Here's how the part is built. I have some questions about the finished solid (model axes, mm). A direction names the side the tool comes from. Coordinates: 2 decimals unless noted, no trailing zeros. Order: outer loops, then holes, each group sorted by start corner. A loop starts at its lowest first (then second) coordinate and runs counter-clockwise, first axis right, second up. Notation, with made-up numbers: (12.5, 35.5) - (42.5, 35.5) arc R16 ccw to (42.5, 44.5) - close; hole circle Ø9 at (-3, 47). An arc over 180 degrees is marked (long way). Answer as CSV lines item,"result". Start each with the question number.
Q1. I need wall thicknesses on line 1 (Y direction, x = 26.5, z = 4); line 2 (X direction, y = 78, z = 1.15); line 3 (Y direction, x = 86, z = 4). Which ranges of each line are inside material? Lowest first, please.
Q2. Suppose I cut it at A-A (x = 50). Please give me the cut outline in (y, z), then the cut area to 4 significant figures.
Q3. For pin 1 Ø2.5 at (y, z) = (35.5, 3.5) entering from +X; pin 2 Ø2.5 at (y, z) = (37.5, 1.5) entering from -X; pin 3 Ø1 at (x, z) = (-26.5, 3.5) entering from -Y, each with a flat end and sliding along its axis, tell me the tip position at first contact or that it passes through.
Q4. Suppose I cut it at B-B (y = -114.5). Please give me the cut outline in (x, z), then the cut area to 3 significant figures.
Q5. Suppose I cut it at D-D (z = 3.95). Count the separate pieces of the cut face and the enclosed holes in it, then the cut area to 3 significant figures.
Q6. For faces 1 (the face through (-3, -86, 0)), 2 (the face through (-78, -44, 3)), 3 (the face through (-67.3, -102.615, 2.535)), which set-ups out of +Z, -Z, +X, -X, +Y, -Y let a thin tool reach every point of the face, with its end or its side?
Q7. Suppose I cut it at C-C (y = -141.5). Please give me the cut outline in (x, z), then the cut area to 3 significant figures.
Q8. Thinking about a two-plate mould opening in X: for faces 4 (the face through (226.035, -75.128, 2.465)), 5 (the face through (67.15, -102.48, 2.54)), 6 (the face through (-225.212, -72.74, 2.465)), which applies, released by +X, released by -X, zero draft, split by the parting line, or undercut?
from build123d import *

# Parameters (mm, degrees)
EXTRUDE_1_OUTLINE_R = 6.05
EXTRUDE_1_DEPTH     = 5
SKETCH_3_R          = 21.1
CUT_EXTRUDE_2_DEPTH = 281.223125384
FILLET_1_R          = 10
FILLET1_R           = 10
CUT_EXTRUDE1_DEPTH  = 10
FILLET2_R           = 5


# Read off the part's stored shape, not the designer's step: 凸台-拉伸1
with BuildPart() as part:
    # 凸台-拉伸1 outline → 凸台-拉伸1 (new body)
    with BuildSketch(Plane.XY):
        with BuildLine():
            ThreePointArc((-97.084973779, -160), (-77.084973779, -132.915026221), (-70, -100))
            Line((-70, -100), (70, -100))
            ThreePointArc((70, -100), (77.084973779, -132.915026221), (97.084973779, -160))
            Line((97.084973779, -160), (202.915026221, -160))
            ThreePointArc((202.915026221, -160), (224.833147735, -71.715728753), (150, -20))
            Line((150, -20), (150, 100))
            Line((150, 100), (-150, 100))
            Line((-150, 100), (-150, -20))
            ThreePointArc((-150, -20), (-224.833147735, -71.715728753), (-202.915026221, -160))
            Line((-202.915026221, -160), (-97.084973779, -160))
        make_face()
        with Locations((-50, -80)):
            Circle(EXTRUDE_1_OUTLINE_R, mode=Mode.SUBTRACT)
        with Locations((50, -80)):
            Circle(EXTRUDE_1_OUTLINE_R, mode=Mode.SUBTRACT)
        with Locations((-130, 0)):
            Circle(EXTRUDE_1_OUTLINE_R, mode=Mode.SUBTRACT)
        with Locations((-130, 79.62392947)):
            Circle(EXTRUDE_1_OUTLINE_R, mode=Mode.SUBTRACT)
        with Locations((130, 0)):
            Circle(EXTRUDE_1_OUTLINE_R, mode=Mode.SUBTRACT)
        with Locations((130, 80)):
            Circle(EXTRUDE_1_OUTLINE_R, mode=Mode.SUBTRACT)
    extrude(amount=EXTRUDE_1_DEPTH)

    # 草图3 → 切除-拉伸2 (cut, through all)
    with BuildSketch(Plane.XY.offset(5)):
        with Locations((-150, -100)):
            Circle(SKETCH_3_R)
        with Locations((150, -100)):
            Circle(SKETCH_3_R)
    extrude(amount=-CUT_EXTRUDE_2_DEPTH, mode=Mode.SUBTRACT)

    # 圆角1
    fillet_1_edges = [part.edges().sort_by_distance(p)[0] for p in [
        (-150, -20, 2.5),
        (-150, 100, 2.5),
        (150, 100, 2.5),
        (150, -20, 2.5),
        (70, -100, 2.5),
        (-70, -100, 2.5),
    ]]
    fillet(fillet_1_edges, radius=FILLET_1_R)

    # Fillet1
    fillet1_edges = [part.edges().sort_by_distance(p)[0] for p in [
        (-97.084973779, -160, 2.5),
        (-202.915026221, -160, 2.5),
        (202.915026221, -160, 2.5),
        (97.084973779, -160, 2.5),
    ]]
    fillet(fillet1_edges, radius=FILLET1_R)

    # Sketch3 → Cut-Extrude1 (cut)
    with BuildSketch(Plane.XY.offset(5)):
        Polygon((-90, 70), (-40, 50), (40, 50), (90, 70), (60, 85), (-60, 85), align=None)
        Polygon((-110, 50), (-110, 20), (-50, 30), align=None)
        Polygon((50, 30), (110, 20), (110, 50), align=None)
        Polygon((-25, 30), (25, 30), (20, -80), (-20, -80), align=None)
        Polygon((-90, 0), (-50, -30), (-110, -60), align=None)
        Polygon((50, -30), (90, 0), (110, -60), align=None)
    extrude(amount=-CUT_EXTRUDE1_DEPTH, mode=Mode.SUBTRACT)

    # Fillet2
    fillet2_edges = [part.edges().sort_by_distance(p)[0] for p in [
        (-110, -60, 2.5),
        (-90, 0, 2.5),
        (-50, -30, 2.5),
        (50, 30, 2.5),
        (110, 50, 2.5),
        (110, 20, 2.5),
        (-110, 50, 2.5),
        (-50, 30, 2.5),
        (-110, 20, 2.5),
        (-20, -80, 2.5),
        (-25, 30, 2.5),
        (25, 30, 2.5),
        (20, -80, 2.5),
        (110, -60, 2.5),
        (50, -30, 2.5),
        (90, 0, 2.5),
        (-90, 70, 2.5),
        (-60, 85, 2.5),
        (60, 85, 2.5),
        (90, 70, 2.5),
        (40, 50, 2.5),
        (-40, 50, 2.5),
    ]]
    fillet(fillet2_edges, radius=FILLET2_R)


solid = part.part
Here are the results:
1,line 1,"y = -100 to 50, 85 to 100"
1,line 2,"x = -150 to -135.83, -124.17 to -74, 74 to 124.29, 135.71 to 150"
1,line 3,"y = -148 to -48, -3.38 to 24, 42 to 100"
2,outline,"(-100, 0) - (-86.05, 0) - (-86.05, 5) - (-100, 5) - close; (-73.95, 0) - (54, 0) - (54, 5) - (-73.95, 5) - close; (85, 0) - (100, 0) - (100, 5) - (85, 5) - close"
2,area,"784.5 mm²"
3,pin 1,"stops at x = 150"
3,pin 2,"stops at x = -150"
3,pin 3,"stops at y = -100"
4,outline,"(-228.67, 0) - (-165.33, 0) - (-165.33, 5) - (-228.67, 5) - close; (-134.67, 0) - (-71.33, 0) - (-71.33, 5) - (-134.67, 5) - close; (71.33, 0) - (134.67, 0) - (134.67, 5) - (71.33, 5) - close; (165.33, 0) - (228.67, 0) - (228.67, 5) - (165.33, 5) - close"
4,area,"1,270 mm²"
5,separate pieces,"1"
5,enclosed holes,"14"
5,area,"69,600 mm²"
6,face 1,"-Z, +X, -X, +Y, -Y"
6,face 2,"+Z, -Z"
6,face 3,"+Z, -Z, -Y"
7,outline,"(-218.39, 0) - (-81.61, 0) - (-81.61, 5) - (-218.39, 5) - close; (81.61, 0) - (218.39, 0) - (218.39, 5) - (81.61, 5) - close"
7,area,"1,370 mm²"
8,face 4,"released by +X"
8,face 5,"undercut"
8,face 6,"released by -X"
